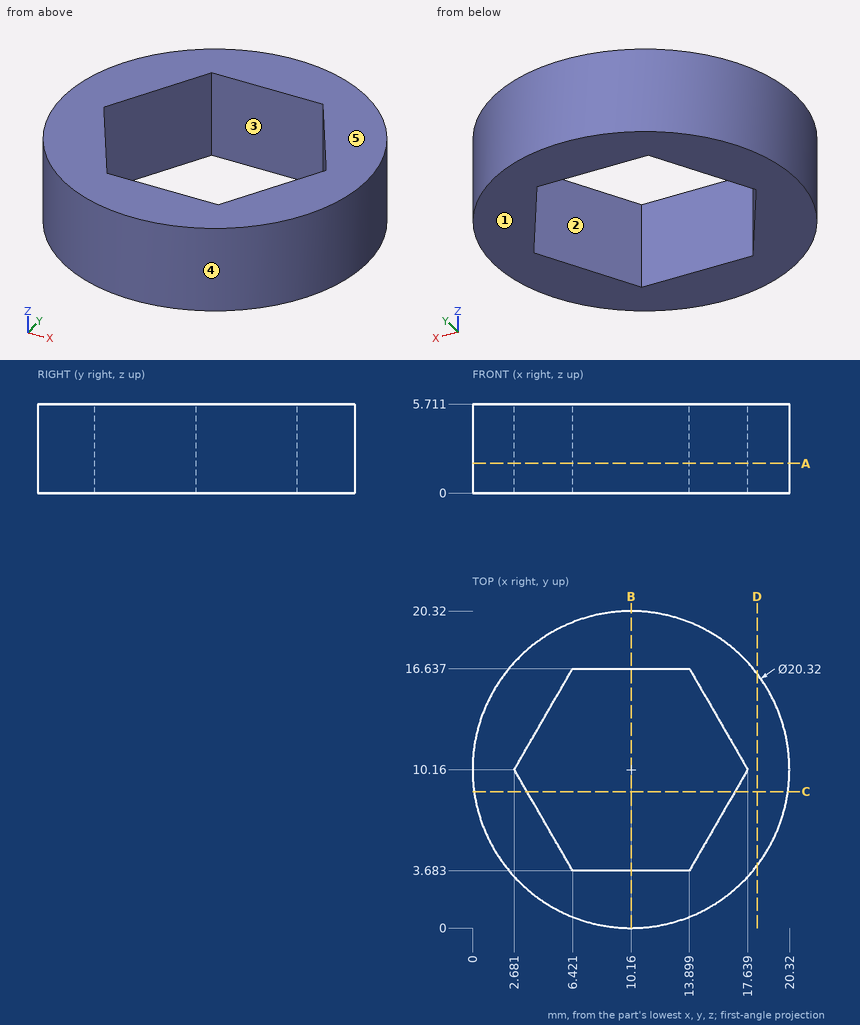
Could you check a few things on this drawing? It's one solid part, dimensions in mm from its lowest x, y, z. A direction names the side the tool comes from. Round coordinates to 2 decimals unless told otherwise and drop trailing zeros. Loops run counter-clockwise (first coordinate to the right, second up) from the corner with the lowest first, then second, coordinate; pieces in that order, holes last.
Q1. I want a section at D-D (x = 18.25). Write out the boundary of the cut face in (y, z).
Q2. Thinking about a two-plate mould opening in X: for the marked faces 3, 4 and 5, which applies, pulls with the +X half, pulls with the -X half, needs draft (parallel to the pull), parting line crosses it, or undercut?
Q3. Please list where these lines run through material, in increasing order: L1, parallel to X at y = 16.5, z = 1.6; L2, parallel to X at y = 10, z = 0.5 (1 decimal); L3, parallel to Y at x = 7.25, z = 1.75 (1 decimal).
Q4. On a 3-axis mill with a long thin cutter (end or side, diameter ignored), from which of +Z, -Z, +X, -X, +Y, -Y can I reach the whole of each face in a straight line? I mean the marked faces 1 and 2. Say none if no direction works.
Q5. For P1, Ø1.5, axis at y = 16.5, z = 4.5, coming from the -X side (1 decimal); P2, Ø3, axis at x = 13, z = 1.5, coming from the -Y side; P3, Ø3, axis at y = 13.5, z = 5, coming from the +X side, each with a flat end and sliding along its axis, tell me the tip position at first contact or that it passes through.
Q6. I want a section at C-C (y = 8.75). Write out the boundary of the cut face in (x, z) (1 decimal), and give its area (3 significant figures).
Q7. I want a section at B-B (x = 10.16). Write out the boundary of the cut face in (y, z).
Q8. I want a section at A-A (z = 1.9). Write out the boundary of the cut face in (x, y), and give its area (3 significant figures).
Answer below:
1. outline: (4.01, 0) - (16.31, 0) - (16.31, 5.71) - (4.01, 5.71) - close
2. face 3: undercut
2. face 4: parting line crosses it
2. face 5: needs draft
3. L1: x = 2.22 to 6.34, 13.98 to 18.1
3. L2: x = 0 to 2.8, 17.5 to 20.3
3. L3: y = 0.4 to 3.7, 16.6 to 19.9
4. face 1: -Z, +X, -X, +Y, -Y
4. face 2: +Z, -Z
5. P1: stops at x = 1.7
5. P2: stops at y = 0.09
5. P3: stops at x = 20.15
6. outline: (0.1, 0) - (3.5, 0) - (3.5, 5.7) - (0.1, 5.7) - close; (16.8, 0) - (20.2, 0) - (20.2, 5.7) - (16.8, 5.7) - close
6. area: 38.8 mm2
7. outline: (0, 0) - (3.68, 0) - (3.68, 5.71) - (0, 5.71) - close; (16.64, 0) - (20.32, 0) - (20.32, 5.71) - (16.64, 5.71) - close
8. outline: circle Ø20.32 at (10.16, 10.16); hole (2.68, 10.16) - (6.42, 3.68) - (13.9, 3.68) - (17.64, 10.16) - (13.9, 16.64) - (6.42, 16.64) - close
8. area: 179 mm2
